Study the drawing (mm; zero at the part's minimum x, y, z) and answer. A direction names the side the tool comes from. Coordinates: 2 decimals unless noted, no trailing zeros. Loops run counter-clockwise (first coordinate to the right, second up) from the corner with the lowest first, then second, coordinate; pieces in that order, holes last. Notation, with made-up numbers: M 40.25,-37.75 L 59.25,-37.75 A16 ccw 59.25,-11.75 Z; hole C 23.25,-37.75 d7. An arc over 180 degrees is marked long. Use one line per item in the form item = value. Start each with the question number.
1. The part is cut by section C-C (x = 24.5). Give the vertices of the cut face in (y, z) (3 decimals).
2. The part is cut by section A-A (z = 18.25). Give the vertices of the cut face in (x, y).
3. For a pull along X with two mould halves and no side action, classify the marked faces 1, 2 and 3 as released by +X, released by -X, zero draft, split by the parting line, or undercut.
4. Find the intervals of material crossed by probe 1 along Z at (x, y) = (13, 13.5); probe 2 along X at (y, z) = (15.5, 12) (1 decimal); probe 3 along Y at (x, z) = (43, 8), in increasing order. Write a range as [from, to].
5. Flat-ended cylindrical pins translate along their axes: pin 1 (3 mm diameter, centred on x = 30, z = 7.5, fed in from -Y); pin 2 (8.5 mm diameter, centred on x = 43.5, z = 12, fed in from -Y); pin 3 (1 mm diameter, centred on y = 10, z = 10, fed in from +X). Find the tip coordinate at first contact, or state that the pin passes through.
6. The part is cut by section B-B (y = 16). Give the number of separate pieces and of enclosed holes in the cut face, plus the area to 3 significant figures.
7. A tool of negligible diameter and unlimited length cuts with its end or side. For the marked faces 4, 5, 6, 7 and 8, from which of +Z, -Z, +X, -X, +Y, -Y can it reach the whole face along a straight path? Write none if from no direction.
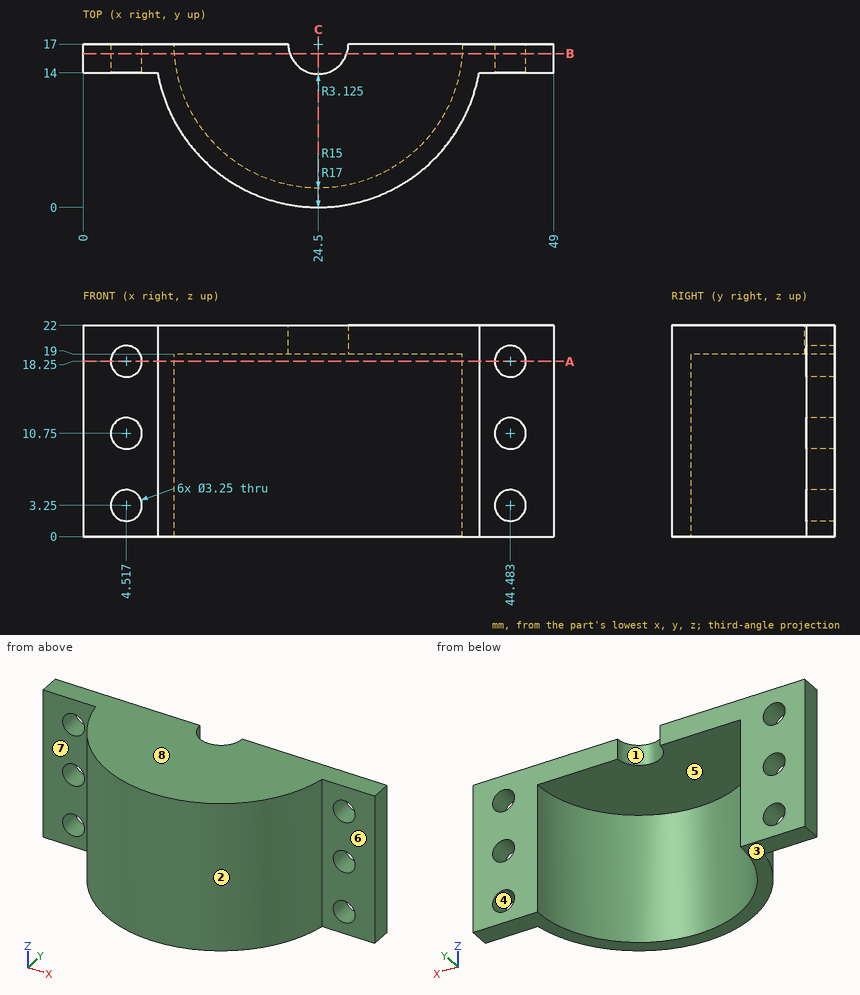
Computed values:
q1.outline = M 0,0 L 2,0 L 2,19 L 13.875,19 L 13.875,22 L 0,22 Z
q2.outline = M 0,14 L 2.89,14 L 2.89,17 L 0,17 Z; M 6.14,14 L 7.77,14 A17 ccw 41.23,14 L 42.86,14 L 42.86,17 L 39.5,17 A15 cw 9.5,17 L 6.14,17 Z; M 46.11,14 L 49,14 L 49,17 L 46.11,17 Z
q3.face_1 = undercut
q3.face_2 = split by the parting line
q3.face_3 = zero draft
q4.probe_1 = [19, 22]
q4.probe_2 = [0, 3.5], [5.6, 9.6], [39.4, 43.4], [45.5, 49]
q4.probe_3 = [14, 17]
q5.pin_1 = 0.48
q5.pin_2 = 8.55
q5.pin_3 = 40.21
q6.separate_pieces = 2
q6.enclosed_holes = 6
q6.area = 442 mm²
q7.face_4 = +Y, -Y
q7.face_5 = -Z, +Y
q7.face_6 = +Z, -Z, +X, -Y
q7.face_7 = +Z, -Z, -X, -Y
q7.face_8 = +Z, +X, -X, +Y, -Y
